from build123d import *

# Parameters (mm, degrees)
SKETCH1_R                       = 80
BOSS_EXTRUDE1_DEPTH             = 5
F_3_0MM_DOWEL_HOLE1_D           = 3
F_3_0MM_DOWEL_HOLE1_DEPTH       = 7.5
F_3_0MM_DOWEL_HOLE1_CSINK_D     = 3.05
F_3_0MM_DOWEL_HOLE1_CSINK_ANGLE = 90
F_3_0MM_DOWEL_HOLE1_TIP         = 0.901290929


with BuildPart() as part:
    # Sketch1 → Boss-Extrude1 (new body)
    with BuildSketch(Plane.XY):
        Polygon((-145, 115), (-115, 145), (115, 145), (145, 115), (145, -115), (115, -145), (-115, -145), (-145, -115), align=None)
        Circle(SKETCH1_R, mode=Mode.SUBTRACT)
    extrude(amount=BOSS_EXTRUDE1_DEPTH)

    # Ø3.0mm Dowel Hole1
    with Locations(Plane.XY.offset(5)):
        with Locations((0, 130), (130, 0), (0, -130), (-130, 0)):
            CounterSinkHole(F_3_0MM_DOWEL_HOLE1_D / 2, F_3_0MM_DOWEL_HOLE1_CSINK_D / 2, depth=F_3_0MM_DOWEL_HOLE1_DEPTH, counter_sink_angle=F_3_0MM_DOWEL_HOLE1_CSINK_ANGLE)
            with Locations((0, 0, -(F_3_0MM_DOWEL_HOLE1_DEPTH + F_3_0MM_DOWEL_HOLE1_TIP / 2))):  # 118° drill point
                Cone(0, F_3_0MM_DOWEL_HOLE1_D / 2, F_3_0MM_DOWEL_HOLE1_TIP, mode=Mode.SUBTRACT)


solid = part.part
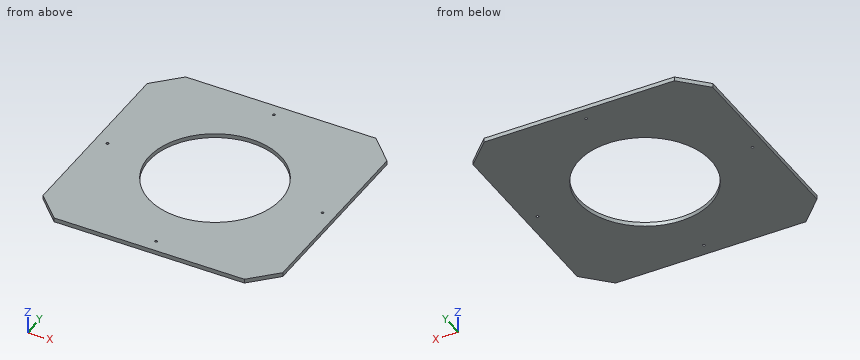
Read the model definition and answer for the solid it produces. Units are mm, in the model's axes. Coordinates: 2 decimals unless noted, no trailing zeros. Write each loop counter-clockwise with the first axis right and the second up, starting at its lowest first coordinate (ties: lowest second). Pieces come first, ordered by that corner, then holes. Notation, with made-up numbers: (27.5, 6.5) - (79.5, 6.5) arc R23 ccw to (79.5, 17.5) - close; hole circle Ø6 at (10, 26.5). An arc over 180 degrees is marked (long way). One line per question, with ' | ' between items.
Q1. This flat-tipped pin is pushed along its axis until it touches: P1, Ø1.8, axis at x = 0, y = 130, coming from the +Z side. Where does it stop, or does it pass through?
Result set:
P1: through
Q2. Consider L1, parallel to Y at x = 0, z = 1.1; L2, parallel to X at y = 62.5, z = 2.3; L3, parallel to Y at x = 52.5, z = 1.7. Determine where each line is inside the solid, lowest interval first. Write a range as [from, to].
Result set:
L1: [-145, -131.5], [-128.5, -80], [80, 128.5], [131.5, 145] | L2: [-145, -49.94], [49.94, 145] | L3: [-145, -60.36], [60.36, 145]
Q3. Find section B-B, the plane y = -37.5. Write down the section's boundary in (x, z), plus the area to 3 significant figures.
Result set:
outline: (-145, 0) - (-70.67, 0) - (-70.67, 5) - (-145, 5) - close; (70.67, 0) - (145, 0) - (145, 5) - (70.67, 5) - close | area: 743 mm^2
Q4. Find section C-C, the plane x = 55.5. Write down the section's boundary in (y, z), plus the area to 3 significant figures.
Result set:
outline: (-145, 0) - (-57.62, 0) - (-57.62, 5) - (-145, 5) - close; (57.62, 0) - (145, 0) - (145, 5) - (57.62, 5) - close | area: 874 mm^2
Q5. Find section A-A, the plane z = 1.35. Write down the section's boundary in (x, y), plus the area to 3 significant figures.
Result set:
outline: (-145, -115) - (-115, -145) - (115, -145) - (145, -115) - (145, 115) - (115, 145) - (-115, 145) - (-145, 115) - close; hole circle Ø3 at (-130, 0); hole circle Ø160 at (0, 0); hole circle Ø3 at (0, -130); hole circle Ø3 at (0, 130); hole circle Ø3 at (130, 0) | area: 62,200 mm^2
